Autodesk Inventor part; units mm, degrees
ref_plane "YZ Plane" through (0, 0, 0) normal (1, 0, 0) x (0, 1, 0)
ref_plane "XZ Plane" through (0, 0, 0) normal (0, 1, 0) x (-1, 0, 0)
ref_plane "XY Plane" through (0, 0, 0) normal (0, 0, 1) x (1, 0, 0)
sketch "Sketch3" plane through (0, 0, 0) normal (1, 0, 0) x (0, 1, 0)
  arc A0 (1.2, 2.3065) -> (-1.2, 2.3065) centre (0, 0) ccw
  line L0 (2.6, 1.2) -> (1.2, 1.2)
  line L1 (1.2, 1.2) -> (1.2, 2.6)
  line L2 (-1.2, 2.6) -> (-1.2, 1.2)
  line L3 (-1.2, 1.2) -> (-2.6, 1.2)
  line L4 (-2.6, -1.2) -> (-1.2, -1.2)
  line L5 (-1.2, -1.2) -> (-1.2, -2.6)
  line L6 (1.2, -2.6) -> (1.2, -1.2)
  line L7 (1.2, -1.2) -> (2.6, -1.2)
  arc A1 (-2.3065, 1.2) -> (-2.3065, -1.2) centre (0, 0) ccw
  arc A2 (-1.2, -2.3065) -> (1.2, -2.3065) centre (0, 0) ccw
  arc A3 (2.3065, -1.2) -> (2.3065, 1.2) centre (0, 0) ccw
  circle A4 centre (0, 0) radius 3.175
  dimension "d31" = 360
  dimension "d36" = 6.35
extrude "Extrusion3" add sketch "Sketch3" along normal blind 5
sketch "Sketch5" plane through (5, 0, 0) normal (1, 0, 0) x (0, 0, -1)
  circle A0 centre (0, 0) radius 2.6
  circle A1 centre (0, 0) radius 10
  dimension "d53" = 20
extrude "Extrusion4" add sketch "Sketch5" against normal blind 2
sketch "Sketch8" plane through (3, 0, 0) normal (-1, 0, 0) x (0, 0, 1)
  circle A0 centre (0, 0) radius 5
  circle A1 centre (0, 0) radius 5.5
  circle A2 centre (0, 0) radius 6.5
  circle A3 centre (0, 0) radius 7
  circle A4 centre (0, 0) radius 8
  circle A5 centre (0, 0) radius 8.5
  dimension "d54" = 10
  dimension "d55" = 11
  dimension "d56" = 13
  dimension "d57" = 14
  dimension "d58" = 16
  dimension "d59" = 17
extrude "Extrusion6" cut sketch "Sketch8" against normal blind 0.1
properties part number "omni-caster-lego-adaptor"
Source: CAD feature listing. Evaluate the final solid. Frame: model axes, mm. A direction names the side the tool comes from. Coordinates: 2 decimals unless noted, no trailing zeros. Loops run counter-clockwise (first coordinate to the right, second up) from the corner with the lowest first, then second, coordinate; pieces in that order, holes last. Notation, with made-up numbers: M 36,9.25 L 44,9.25 A13 cw 44,32.25 Z; hole C -34,70 d2. An arc over 180 degrees is marked long. Use a Markdown table: item, result. Add a question column.
Q1. Access query for faces 4 (the cylindrical face through (2.5, 2.6, 0)), 5 (the flat face through (3, 3, 5)), 6 (the flat face through (0, 1.4, -1.4)). Directions: +Z, -Z, +X, -X, +Y, -Y. A direction counts if a zero-diameter tool reaches every point of the face in a straight line with its end or side. Return the directions, or none.
Q2. Section query A-A, the plane y = -4.5. Return loops of the section in (x, z), and give its area (3 significant figures).
Q3. Section query D-D, the plane z = 7.75. Return loops of the section in (x, y), and give its area (3 significant figures).
Q4. Draft query along Y for faces 1 (the flat face through (3.1, -4.9, 1.6)), 2 (the cylindrical face through (1.48, -0.69, 3.1)), 3 (the flat face through (3, -7.4, 4.5)). Return one class per face: pulls with the +Y half, pulls with the -Y half, needs draft (parallel to the pull), parting line crosses it, or undercut.
Q5. Section query B-B, the plane z = 4. Return loops of the section in (x, y), and give its area (3 significant figures).
Q6. First-contact query: pin 1 (6.5 mm diameter, centred on y = 0, z = 0, fed in from +X); pin 2 (1.5 mm diameter, centred on x = 1.5, z = -0.5, fed in from +Y) (3 decimals); pin 3 (0.6 mm diameter, centred on x = 3.5, y = -1.5, fed in from +Z); pin 4 (0.9 mm diameter, centred on x = 2.5, z = -2, fed in from -Y). Flat tips, straight axial feed; report the tip coordinate or a pass-through.
Q7. Section query C-C, the plane z = -5.25. Return loops of the section in (x, y), and give its area (3 significant figures).
Q8. Material intervals for L1, parallel to X at y = -6, z = -1.75; L2, parallel to Y at x = 4.25, z = -6; L3, parallel to X at y = 1.75, z = 6.5, sorted ascending.
Result:
| question | item | result |
|---|---|---|
| 1 | face 4 | +X, -X |
| 1 | face 5 | -X |
| 1 | face 6 | +Z, -Z, -X, +Y, -Y |
| 2 | outline | M 3,-8.93 L 5,-8.93 L 5,8.93 L 3,8.93 L 3,7.21 L 3.1,7.21 L 3.1,6.61 L 3,6.61 L 3,5.36 L 3.1,5.36 L 3.1,4.69 L 3,4.69 L 3,3.16 L 3.1,3.16 L 3.1,2.18 L 3,2.18 L 3,-2.18 L 3.1,-2.18 L 3.1,-3.16 L 3,-3.16 L 3,-4.69 L 3.1,-4.69 L 3.1,-5.36 L 3,-5.36 L 3,-6.61 L 3.1,-6.61 L 3.1,-7.21 L 3,-7.21 Z |
| 2 | area | 35.3 mm2 |
| 3 | outline | M 3,-6.32 L 5,-6.32 L 5,6.32 L 3,6.32 L 3,3.49 L 3.1,3.49 L 3.1,1.98 L 3,1.98 L 3,-1.98 L 3.1,-1.98 L 3.1,-3.49 L 3,-3.49 Z |
| 3 | area | 25.0 mm2 |
| 4 | face 1 | undercut |
| 4 | face 2 | parting line crosses it |
| 4 | face 3 | needs draft |
| 5 | outline | M 3,-9.17 L 5,-9.17 L 5,9.17 L 3,9.17 L 3,7.5 L 3.1,7.5 L 3.1,6.93 L 3,6.93 L 3,5.74 L 3.1,5.74 L 3.1,5.12 L 3,5.12 L 3,3.77 L 3.1,3.77 L 3.1,3 L 3,3 L 3,-3 L 3.1,-3 L 3.1,-3.77 L 3,-3.77 L 3,-5.12 L 3.1,-5.12 L 3.1,-5.74 L 3,-5.74 L 3,-6.93 L 3.1,-6.93 L 3.1,-7.5 L 3,-7.5 Z |
| 5 | area | 36.3 mm2 |
| 6 | pin 1 | stops at x = 5 |
| 6 | pin 2 | stops at y = 3.175 |
| 6 | pin 3 | stops at z = 9.93 |
| 6 | pin 4 | stops at y = -2.77 |
| 7 | outline | M 3,-8.51 L 5,-8.51 L 5,8.51 L 3,8.51 L 3,6.68 L 3.1,6.68 L 3.1,6.04 L 3,6.04 L 3,4.63 L 3.1,4.63 L 3.1,3.83 L 3,3.83 L 3,1.64 L 3.1,1.64 L 3.1,-1.64 L 3,-1.64 L 3,-3.83 L 3.1,-3.83 L 3.1,-4.63 L 3,-4.63 L 3,-6.04 L 3.1,-6.04 L 3.1,-6.68 L 3,-6.68 Z |
| 7 | area | 33.4 mm2 |
| 8 | L1 | x = 3 to 5 |
| 8 | L2 | y = -8 to 8 |
| 8 | L3 | x = 3.1 to 5 |
